Input: dimensioned drawing with shaded views. Units: mm. Origin: part minimum x, y, z. A direction names the side the tool comes from. Round coordinates to 2 decimals unless told otherwise and drop trailing zeros. Loops run counter-clockwise (first coordinate to the right, second up) from the corner with the lowest first, then second, coordinate; pieces in that order, holes last. Notation, with made-up numbers: M -8,70 L 5,70 A21 ccw 5,102 Z; hole C 48.5,69.5 d1. An arc over 180 degrees is marked long. Return JSON: item names as keys, results as strings.
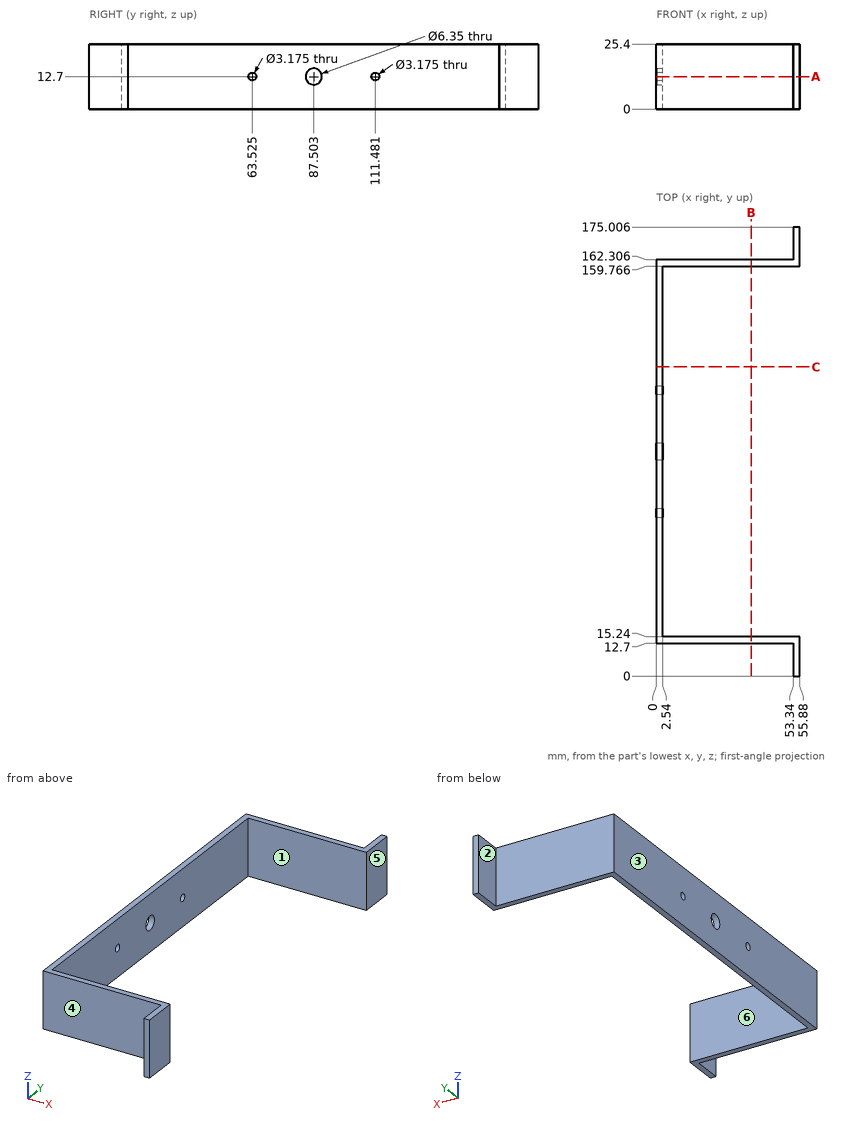
Q1. Section query B-B (x = 37). Output: boundary loops of the cut face in (y, z).
Determined:
{"outline": "M 12.7,0 L 15.24,0 L 15.24,25.4 L 12.7,25.4 Z; M 159.77,0 L 162.31,0 L 162.31,25.4 L 159.77,25.4 Z"}
Q2. Material intervals for L1, parallel to Y at x = 15.5, z = 10.5; L2, parallel to X at y = 142, z = 19.25; L3, parallel to X at y = 7, z = 17.5, sorted ascending.
Determined:
{"L1": "y = 12.7 to 15.24, 159.77 to 162.31", "L2": "x = 0 to 2.54", "L3": "x = 53.34 to 55.88"}
Q3. Section query A-A (z = 12.7). Output: boundary loops of the cut face in (x, y).
Determined:
{"outline": "M 0,12.7 L 53.34,12.7 L 53.34,0 L 55.88,0 L 55.88,15.24 L 2.54,15.24 L 2.54,61.94 L 0,61.94 Z; M 0,65.11 L 2.54,65.11 L 2.54,84.33 L 0,84.33 Z; M 0,90.68 L 2.54,90.68 L 2.54,109.89 L 0,109.89 Z; M 0,113.07 L 2.54,113.07 L 2.54,159.77 L 55.88,159.77 L 55.88,175.01 L 53.34,175.01 L 53.34,162.31 L 0,162.31 Z"}
Q4. Pin query (flat end, axial travel): pin 1 (12.5 mm diameter, centred on x = 17, z = 18, fed in from +Y); pin 2 (1.5 mm diameter, centred on y = 116, z = 12.5, fed in from +X); pin 3 (4 mm diameter, centred on y = 3.5, z = 12.5, fed in from -X). Return the tip coordinate at first contact, or that it passes through.
Determined:
{"pin 1": "stops at y = 162.31", "pin 2": "stops at x = 2.54", "pin 3": "stops at x = 53.34"}
Q5. Pull-direction query (Y, two-part tool) for the marked faces 4, 5 and 6; classes: pulls with the +Y half, pulls with the -Y half, needs draft (parallel to the pull), parting line crosses it, or undercut.
Determined:
{"face 4": "pulls with the -Y half", "face 5": "needs draft", "face 6": "undercut"}
Q6. Reachability of the marked faces 1, 2 and 3 from +Z, -Z, +X, -X, +Y, -Y: full face, straight path, thin tool, end or side. Return the list, or none.
Determined:
{"face 1": "+Z, -Z, +X", "face 2": "+Z, -Z, -X, +Y", "face 3": "+Z, -Z, -X, +Y, -Y"}
Q7. Section query C-C (y = 120.5). Output: boundary loops of the cut face in (x, z).
Determined:
{"outline": "M 0,0 L 2.54,0 L 2.54,25.4 L 0,25.4 Z"}
